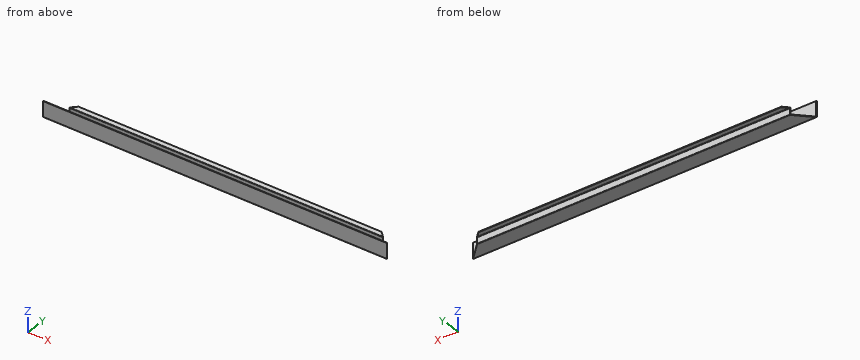
```python
from build123d import *

# Parameters (mm, degrees)
BOSS_EXTRUDE1_DEPTH = 1930
FILLET1_R           = 3
CUT_EXTRUDE1_DEPTH  = 88
CUT_EXTRUDE2_DEPTH  = 88


with BuildPart() as part:
    # Sketch1 → Boss-Extrude1 (new body)
    with BuildSketch(Plane(origin=(0, 0, 0), x_dir=(0, 0, -1), z_dir=(1, 0, 0))):
        Polygon((0, 0), (85, 0), (85, 82), (47, 82), (47, 112), (50, 112), (50, 85), (88, 85), (88, -3), (0, -3), align=None)
    extrude(amount=BOSS_EXTRUDE1_DEPTH)

    # Fillet1
    fillet1_edges = [part.edges().sort_by_distance(p)[0] for p in [
        (965, 0, -85),
        (965, 82, -85),
        (965, 82, -47),
        (965, 85, -50),
        (965, 85, -88),
        (965, -3, -88),
    ]]
    fillet(fillet1_edges, radius=FILLET1_R)

    # Sketch4 → Cut-Extrude1 (cut)
    with BuildSketch(Plane(origin=(0, 0, -88), x_dir=(-1, 0, 0), z_dir=(0, 0, -1))):
        Polygon((-1930, -3), (-1815, 112), (-1930, 112), align=None)
    extrude(amount=-CUT_EXTRUDE1_DEPTH, mode=Mode.SUBTRACT)

    # Sketch5 → Cut-Extrude2 (cut)
    with BuildSketch(Plane(origin=(0, 0, -88), x_dir=(-1, 0, 0), z_dir=(0, 0, -1))):
        Polygon((0, -3), (-115, 112), (0, 112), align=None)
    extrude(amount=-CUT_EXTRUDE2_DEPTH, mode=Mode.SUBTRACT)


solid = part.part
```
For this review, take the finished solid that the model builds, in its own axes (mm). Round coordinates to 2 decimals unless told otherwise and drop trailing zeros. Write each loop counter-clockwise with the first axis right and the second up, starting at its lowest first coordinate (ties: lowest second). Pieces come first, ordered by that corner, then holes. Notation, with made-up numbers: (72.25, 59.25) -> (102.25, 59.25) arc R32 ccw to (102.25, 94.25) -> close; hole circle Ø9 at (-26.75, -5). An arc over 180 degrees is marked (long way). Use one line per item in the form item = value.
Q1. Consider section B-B (x = 505.5). State the section outline as (y, z) points.
Resolved:
outline = (-3, -85) arc R3 ccw to (0, -88) -> (82, -88) arc R3 ccw to (85, -85) -> (85, -53) arc R3 cw to (88, -50) -> (112, -50) -> (112, -47) -> (85, -47) arc R3 ccw to (82, -50) -> (82, -82) arc R3 cw to (79, -85) -> (3, -85) arc R3 cw to (0, -82) -> (0, 0) -> (-3, 0) -> close
Q2. Consider section A-A (z = -67). State the section outline as (x, y) points, then the cut area to 3 significant figures.
Resolved:
outline = (0, -3) -> (1930, -3) -> (1927, 0) -> (3, 0) -> close; (85, 82) -> (1845, 82) -> (1842, 85) -> (88, 85) -> close
area = 11,100 mm²
Q3. To check wall thickness, follow probe 1 along Y at (x, z) = (1392, -64.5); probe 2 along Z at (x, y) = (179, 18.5); probe 3 along Y at (x, z) = (348, -23). State the ranges of each line that lie inside material, in increasing order. Write a range as from..to.
Resolved:
probe_1 = -3..0, 82..85
probe_2 = -88..-85
probe_3 = -3..0
Q4. Consider section C-C (y = 37.5). State the section outline as (x, z) points.
Resolved:
outline = (40.5, -88) -> (1889.5, -88) -> (1889.5, -85) -> (40.5, -85) -> close
Q5. Clearance check with flat-ended pins moving along their axes: pin 1 Ø13.5 at (x, y) = (1171, 102.5) entering from +Z; pin 2 Ø5 at (x, z) = (1349.5, -58) entering from +Y; pin 3 Ø7 at (x, y) = (578.5, 100) entering from -Z; pin 4 Ø8 at (y, z) = (61.5, -78) entering from +X. State where each tip first meets the part, or that it passes through.
Resolved:
pin_1 = -47
pin_2 = 85
pin_3 = -50
pin_4 = through
